Verification items for this drawing (mm, ordinates from the low corner). A direction names the side the tool comes from. Coordinates: 2 decimals unless noted, no trailing zeros. Order: outer loops, then holes, each group sorted by start corner. A loop starts at its lowest first (then second) coordinate and runs counter-clockwise, first axis right, second up. Notation, with made-up numbers: M 45.5,0 L 96.5,0 A22 cw 96.5,32 Z; hole C 85.25,-36.75 d6. An arc over 180 degrees is marked long. Return JSON: item names as keys, results as strings. Group by question number.
1. Set-up check for the marked faces 1 and 2: record each of +Z, -Z, +X, -X, +Y, -Y from which the full face is reachable in a straight line by a thin tool's end or side.
2. Material ranges on line 1 along Y through (x, z) = (12.8, 9); line 2 along Z through (x, y) = (12.8, 17.05); line 3 along Y through (x, z) = (12.8, 6.25), recorded low to high.
3. Section check A-A, the plane x = 12.8. Record the cut outline in (y, z), plus the area to 3 significant figures.
4. Section check D-D, the plane x = 16.25. Record the cut outline in (y, z), plus the area to 3 significant figures.
5. Section check B-B, the plane y = 12.8. Record the cut outline in (x, z).
6. Mould release check, pull along Z, two halves, no side actions. Record for the marked faces 3, 4 and 5: +Z half, -Z half, draft (parallel to the pull), parting line (faces both ways), or undercut.
7. Section check C-C, the plane z = 5.75. Record the cut outline in (x, y), plus the area to 3 significant figures.
8. Gauge pin test, flat ends, axial feed: pin 1 (2 mm diameter, centred on x = 13.5, z = 4, fed in from +Y); pin 2 (6 mm diameter, centred on x = 17.5, z = 11, fed in from -Y). Record the tip position at first contact, or that the pin passes through.
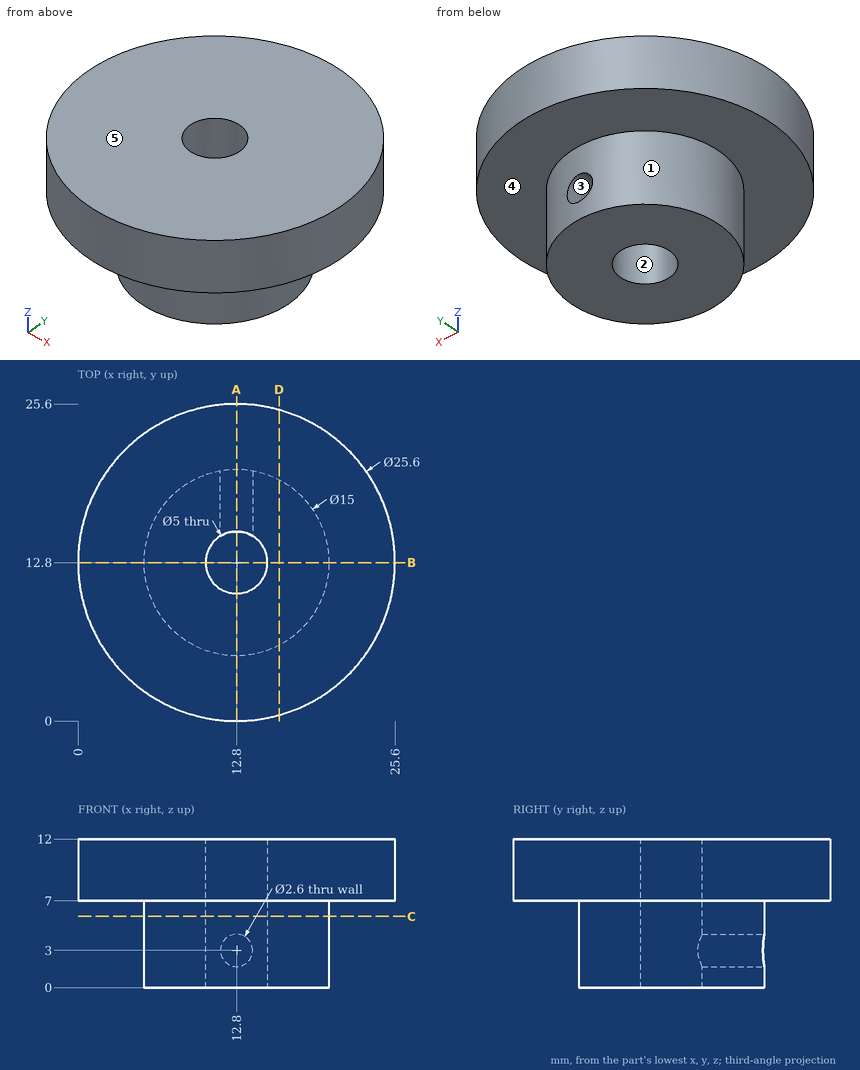
Answers follow:
{
 "1": {"face 1": "-Z", "face 2": "+Z, -Z"},
 "2": {"line 1": "0 to 10.3, 15.3 to 25.6", "line 2": "0 to 1.7, 4.3 to 12", "line 3": "5.3 to 10.3, 15.3 to 20.3"},
 "3": {"outline": "M 0,7 L 5.3,7 L 5.3,0 L 10.3,0 L 10.3,12 L 0,12 Z; M 15.3,0 L 20.3,0 L 20.3,1.7 L 15.3,1.7 Z; M 15.3,4.3 L 20.3,4.3 L 20.3,7 L 25.6,7 L 25.6,12 L 15.3,12 Z", "area": "160 mm^2"},
 "4": {"outline": "M 0.47,7 L 6.14,7 L 6.14,0 L 19.46,0 L 19.46,7 L 25.13,7 L 25.13,12 L 0.47,12 Z", "area": "216 mm^2"},
 "5": {"outline": "M 0,7 L 5.3,7 L 5.3,0 L 10.3,0 L 10.3,12 L 0,12 Z; M 15.3,0 L 20.3,0 L 20.3,7 L 25.6,7 L 25.6,12 L 15.3,12 Z"},
 "6": {"face 3": "undercut", "face 4": "-Z half", "face 5": "+Z half"},
 "7": {"outline": "C 12.8,12.8 d15; hole C 12.8,12.8 d5", "area": "157 mm^2"},
 "8": {"pin 1": "y = 20.3", "pin 2": "y = 0.11"}
}
